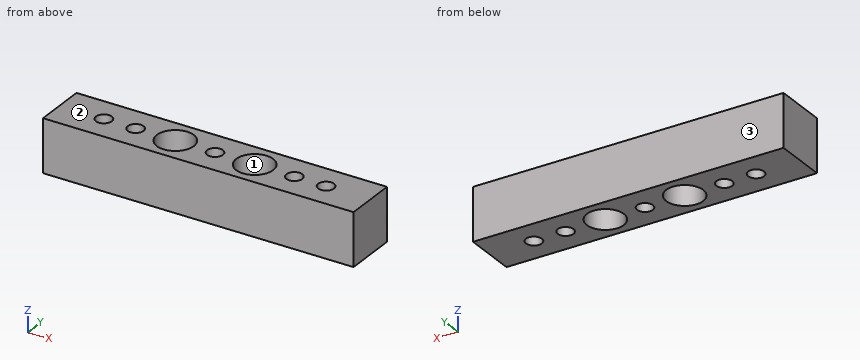
```python
from build123d import *

# Parameters (mm, degrees)
F0_W     = 58.7
F0_H     = 10
F0_R     = 1.5
F0_R_2   = 3.5
F1_DEPTH = 10


with BuildPart() as f1:
    # F0 (on Top) → F1 (new body)
    with BuildSketch(Plane.XY):
        Rectangle(F0_W, F0_H)
        with Locations((-21, 0)):
            Circle(F0_R, mode=Mode.SUBTRACT)
        with Locations((-15, 0)):
            Circle(F0_R, mode=Mode.SUBTRACT)
        with Locations((-7.5, 0)):
            Circle(F0_R_2, mode=Mode.SUBTRACT)
        Circle(F0_R, mode=Mode.SUBTRACT)
        with Locations((7.5, 0)):
            Circle(F0_R_2, mode=Mode.SUBTRACT)
        with Locations((15, 0)):
            Circle(F0_R, mode=Mode.SUBTRACT)
        with Locations((21, 0)):
            Circle(F0_R, mode=Mode.SUBTRACT)
    extrude(amount=F1_DEPTH)


solid = f1.part
```
The listing builds one solid part. Answer for the finished solid, in the listing's coordinates (mm). Face numbers are marked on the shaded views. Give positions to 0.01 mm unless a question says otherwise; leave off trailing zeros. Loops run counter-clockwise (first coordinate to the right, second up) from the corner with the lowest first, then second, coordinate; pieces in that order, holes last. Notation, with made-up numbers: (35.25, 7.5) - (46.25, 7.5) arc R13 ccw to (46.25, 13.5) - close; hole circle Ø2 at (72, 26.5). An arc over 180 degrees is marked (long way). Return JSON: item names as keys, results as strings. Group by question number.
1. Determine the mould class of the marked faces 1, 2 and 3 for opening direction Y: pulls with the +Y half, pulls with the -Y half, needs draft (parallel to the pull), parting line crosses it, or undercut.
2. Find section B-B (z = 7.5). Write down the section's boundary in (x, y).
3. Find section D-D (x = 0). Write down the section's boundary in (y, z).
4. Find section C-C (y = 0). State how many separate pieces and enclosed holes the cut face has, then the cut area to 3 significant figures.
5. Find section A-A (x = 7.5). Write down the section's boundary in (y, z), then the cut area to 3 significant figures.
6. Straight lines are drawn through the part: line 1 (Y direction, x = 0, z = 8); line 2 (X direction, y = -2, z = 3.5); line 3 (X direction, y = 1.75, z = 4.25). For each, find the intervals that lie inside material, in ascending order. Write a range as [from, to].
7. Given pin 1 Ø1.8 at (x, y) = (-15, 0) entering from -Z, flat-ended and moving along its own axis, determine where the tip first touches the part or whether it passes through.
Verdict:
{
 "1": {"face 1": "undercut", "face 2": "needs draft", "face 3": "pulls with the +Y half"},
 "2": {"outline": "(-29.35, -5) - (29.35, -5) - (29.35, 5) - (-29.35, 5) - close; hole circle Ø3 at (-21, 0); hole circle Ø3 at (-15, 0); hole circle Ø7 at (-7.5, 0); hole circle Ø3 at (0, 0); hole circle Ø7 at (7.5, 0); hole circle Ø3 at (15, 0); hole circle Ø3 at (21, 0)"},
 "3": {"outline": "(-5, 0) - (-1.5, 0) - (-1.5, 10) - (-5, 10) - close; (1.5, 0) - (5, 0) - (5, 10) - (1.5, 10) - close"},
 "4": {"separate pieces": "8", "enclosed holes": "0", "area": "297 mm^2"},
 "5": {"outline": "(-5, 0) - (-3.5, 0) - (-3.5, 10) - (-5, 10) - close; (3.5, 0) - (5, 0) - (5, 10) - (3.5, 10) - close", "area": "30.0 mm^2"},
 "6": {"line 1": "y = [-5, -1.5], [1.5, 5]", "line 2": "x = [-29.35, -10.37], [-4.63, 4.63], [10.37, 29.35]", "line 3": "x = [-29.35, -10.53], [-4.47, 4.47], [10.53, 29.35]"},
 "7": {"pin 1": "passes through"}
}
